Geometry check sheet. Reference: the model listing, model coordinates, mm. A direction names the side the tool comes from. Round coordinates to 2 decimals unless told otherwise and drop trailing zeros. Order: outer loops, then holes, each group sorted by start corner. A loop starts at its lowest first (then second) coordinate and runs counter-clockwise, first axis right, second up.
(1) Cross-section at C-C on x = -13. Enter the section's corners in (y, z).
(2) Cross-section at B-B on x = 0. Enter the section's corners in (y, z), and give its area (3 significant figures).
(3) Cross-section at D-D on z = 27. Enter the section's corners in (x, y).
(4) Cross-section at A-A on z = 0. Enter the section's corners in (x, y), and give its area (3 significant figures).
(5) Set-up check for faces 4 (the face through (-17.669, 13.945, 27.714)), 5 (the face through (27.695, 2.129, -21.236)), 6 (the face through (21, 20.066, 26)): record each of +Z, -Z, +X, -X, +Y, -Y from which the full face is reachable in a straight line by a thin tool's end or side.
(6) Draft check along Z on faces 1 (the face through (5.669, 13.393, -1.785)), 2 (the face through (26, 4.318, -21)), 3 (the face through (27.695, 10.003, -21.236)). Enter one of: pulls with the +Z half, pulls with the -Z half, needs draft (parallel to the pull), parting line crosses it, or undercut.
(7) Gauge pin test, flat ends, axial feed: P1, Ø4, axis at y = 11.5, z = 16, coming from the -X side; P2, Ø6, axis at y = 10, z = -9, coming from the +X side; P3, Ø12, axis at x = 26, y = 4.5, coming from the -Z side. Record the tip position at first contact, or that the pin passes through.
(8) Thickness scan on L1, parallel to Z at x = 0, y = 21; L2, parallel to Z at x = 0, y = 8.5; L3, parallel to X at y = 20, z = -14.5. Record the ranges inside material, lowest first.
from build123d import *

# Parameters (mm, degrees)
F_1_4_18_NPSM_TAPPED_HOLE1_D = 11.8872


with BuildPart() as part:
    # Sketch8 → Revolve1 (revolve)
    with BuildSketch(Plane.XY):
        Polygon((0, 0), (0, 26.416), (-33.0835, 26.416), (-33.0835, 20.066), (-34.8996, 20.066), (-34.8996, 15.748), (-32.8676, 15.748), (-32.8676, 12.192), (-34.8996, 12.192), (-34.8996, 7.874), (-32.8676, 7.874), (-32.8676, 4.318), (-34.8996, 4.318), (-34.8996, 0), align=None)
    revolve(axis=Axis((0, 0, 0), (0, 1, 0)))

    # 1/4-18 NPSM Tapped Hole1 (through all)
    with Locations(Plane(origin=(0, 0, 0), x_dir=(-1, 0, 0), z_dir=(0, -1, 0))):
        with Locations((0, 0)):
            Hole(F_1_4_18_NPSM_TAPPED_HOLE1_D / 2)


solid = part.part
Found:
1. outline: (0, -32.39) - (4.32, -32.39) - (4.32, -30.19) - (7.87, -30.19) - (7.87, -32.39) - (12.19, -32.39) - (12.19, -30.19) - (15.75, -30.19) - (15.75, -32.39) - (20.07, -32.39) - (20.07, -30.42) - (26.42, -30.42) - (26.42, 30.42) - (20.07, 30.42) - (20.07, 32.39) - (15.75, 32.39) - (15.75, 30.19) - (12.19, 30.19) - (12.19, 32.39) - (7.87, 32.39) - (7.87, 30.19) - (4.32, 30.19) - (4.32, 32.39) - (0, 32.39) - close
2. outline: (0, -34.9) - (4.32, -34.9) - (4.32, -32.87) - (7.87, -32.87) - (7.87, -34.9) - (12.19, -34.9) - (12.19, -32.87) - (15.75, -32.87) - (15.75, -34.9) - (20.07, -34.9) - (20.07, -33.08) - (26.42, -33.08) - (26.42, -5.94) - (0, -5.94) - close; (0, 5.94) - (26.42, 5.94) - (26.42, 33.08) - (20.07, 33.08) - (20.07, 34.9) - (15.75, 34.9) - (15.75, 32.87) - (12.19, 32.87) - (12.19, 34.9) - (7.87, 34.9) - (7.87, 32.87) - (4.32, 32.87) - (4.32, 34.9) - (0, 34.9) - close
2. area: 1,480 mm2
3. outline: (-22.11, 0) - (22.11, 0) - (22.11, 4.32) - (18.74, 4.32) - (18.74, 7.87) - (22.11, 7.87) - (22.11, 12.19) - (18.74, 12.19) - (18.74, 15.75) - (22.11, 15.75) - (22.11, 20.07) - (19.12, 20.07) - (19.12, 26.42) - (-19.12, 26.42) - (-19.12, 20.07) - (-22.11, 20.07) - (-22.11, 15.75) - (-18.74, 15.75) - (-18.74, 12.19) - (-22.11, 12.19) - (-22.11, 7.87) - (-18.74, 7.87) - (-18.74, 4.32) - (-22.11, 4.32) - close
4. outline: (-34.9, 0) - (-5.94, 0) - (-5.94, 26.42) - (-33.08, 26.42) - (-33.08, 20.07) - (-34.9, 20.07) - (-34.9, 15.75) - (-32.87, 15.75) - (-32.87, 12.19) - (-34.9, 12.19) - (-34.9, 7.87) - (-32.87, 7.87) - (-32.87, 4.32) - (-34.9, 4.32) - close; (5.94, 0) - (34.9, 0) - (34.9, 4.32) - (32.87, 4.32) - (32.87, 7.87) - (34.9, 7.87) - (34.9, 12.19) - (32.87, 12.19) - (32.87, 15.75) - (34.9, 15.75) - (34.9, 20.07) - (33.08, 20.07) - (33.08, 26.42) - (5.94, 26.42) - close
4. area: 1,480 mm2
5. face 4: none
5. face 5: +Y, -Y
5. face 6: +Y
6. face 1: undercut
6. face 2: needs draft
6. face 3: parting line crosses it
7. P1: stops at x = -31.97
7. P2: stops at x = 34.38
7. P3: stops at z = -28.6
8. L1: z = -33.08 to -5.94, 5.94 to 33.08
8. L2: z = -34.9 to -5.94, 5.94 to 34.9
8. L3: x = -31.74 to 31.74
